```python
from build123d import *

# Parameters (mm, degrees)
CROQUIS1_R              = 8.15
CROQUIS1_R_2            = 1.6
SALIENTE_EXTRUIR1_DEPTH = 5
CROQUIS2_R              = 9.1
CORTAR_EXTRUIR1_DEPTH   = 1
CORTAR_EXTRUIR2_DEPTH   = 3
REDONDEO1_R             = 1
SALIENTE_EXTRUIR2_DEPTH = 46
CORTAR_EXTRUIR3_DEPTH   = 2
CORTAR_EXTRUIR4_REACH   = 103.242
CROQUIS6_R              = 2.6
CROQUIS6_W              = 5.6
CROQUIS6_H              = 3
CORTAR_EXTRUIR5_DEPTH   = 5
SALIENTE_EXTRUIR3_DEPTH = 46
CORTAR_EXTRUIR6_DEPTH   = 2
CORTAR_EXTRUIR7_REACH   = 103.242
CROQUIS10_R             = 2.6
CROQUIS10_W             = 5.6
CROQUIS10_H             = 3
CROQUIS11_R             = 1.6
CORTAR_EXTRUIR8_DEPTH   = 21
REDONDEO2_R             = 1


with BuildPart() as part:
    # Croquis1 → Saliente-Extruir1 (new body)
    with BuildSketch(Plane(origin=(0, 0, 0), x_dir=(1, 0, 0), z_dir=(0, 1, 0))):
        with BuildLine():
            Line((-30, -35), (30, -35))
            ThreePointArc((30, -35), (47.67766953, -27.67766953), (55, -10))
            Line((55, -10), (55, 15))
            ThreePointArc((55, 15), (49.142135624, 29.142135624), (35, 35))
            Line((35, 35), (-35, 35))
            ThreePointArc((-35, 35), (-49.142135624, 29.142135624), (-55, 15))
            Line((-55, 15), (-55, -10))
            ThreePointArc((-55, -10), (-47.67766953, -27.67766953), (-30, -35))
        make_face()
        with Locations(Location((39, 9, 0), (0, 0, 270))):
            Circle(CROQUIS1_R, mode=Mode.SUBTRACT)
        with Locations(Location((51.75, 12, 0), (0, 0, 270))):
            Circle(CROQUIS1_R_2, mode=Mode.SUBTRACT)
        with Locations(Location((51.75, -12, 0), (0, 0, 90))):
            Circle(CROQUIS1_R_2, mode=Mode.SUBTRACT)
        with Locations(Location((-51.75, -12, 0), (0, 0, 270))):
            Circle(CROQUIS1_R_2, mode=Mode.SUBTRACT)
        with Locations(Location((-51.75, 12, 0), (0, 0, 90))):
            Circle(CROQUIS1_R_2, mode=Mode.SUBTRACT)
        with Locations(Location((-39, 9, 0), (0, 0, 90))):
            Circle(CROQUIS1_R, mode=Mode.SUBTRACT)
        with BuildLine():
            Line((-10, -23), (10, -23))
            ThreePointArc((10, -23), (17.071067812, -20.071067812), (20, -13))
            Line((20, -13), (20, 13))
            ThreePointArc((20, 13), (17.071067812, 20.071067812), (10, 23))
            Line((10, 23), (-10, 23))
            ThreePointArc((-10, 23), (-17.071067812, 20.071067812), (-20, 13))
            Line((-20, 13), (-20, -13))
            ThreePointArc((-20, -13), (-17.071067812, -20.071067812), (-10, -23))
        make_face(mode=Mode.SUBTRACT)
    extrude(amount=SALIENTE_EXTRUIR1_DEPTH)

    # Croquis2 → Cortar-Extruir1 (cut)
    with BuildSketch(Plane(origin=(0, 5, 0), x_dir=(1, 0, 0), z_dir=(0, 1, 0))):
        with Locations(Location((39, 9, 0), (0, 0, 270))):
            Circle(CROQUIS2_R)
        with Locations(Location((-39, 9, 0), (0, 0, 90))):
            Circle(CROQUIS2_R)
    extrude(amount=-CORTAR_EXTRUIR1_DEPTH, mode=Mode.SUBTRACT)

    # Croquis3 → Cortar-Extruir2 (cut)
    with BuildSketch(Plane(origin=(0, 5, 0), x_dir=(1, 0, 0), z_dir=(0, 1, 0))):
        with BuildLine():
            Line((51.75, 15), (55, 15))
            Line((55, 15), (55, 9))
            Line((55, 9), (51.75, 9))
            ThreePointArc((51.75, 9), (48.75, 12), (51.75, 15))
        make_face()
        with BuildLine():
            Line((51.75, -15), (55, -15))
            Line((55, -15), (55, -9))
            Line((55, -9), (51.75, -9))
            ThreePointArc((51.75, -9), (48.75, -12), (51.75, -15))
        make_face()
        with BuildLine():
            Line((-51.75, -9), (-55, -9))
            Line((-55, -9), (-55, -15))
            Line((-55, -15), (-51.75, -15))
            ThreePointArc((-51.75, -15), (-48.75, -12), (-51.75, -9))
        make_face()
        with BuildLine():
            Line((-51.75, 15), (-55, 15))
            Line((-55, 15), (-55, 9))
            Line((-55, 9), (-51.75, 9))
            ThreePointArc((-51.75, 9), (-48.75, 12), (-51.75, 15))
        make_face()
    extrude(amount=-CORTAR_EXTRUIR2_DEPTH, mode=Mode.SUBTRACT)

    # Redondeo1
    redondeo1_edges = [part.edges().sort_by_distance(p)[0] for p in [
        (-55, 3.5, -9),
        (-55, 3.5, 9),
        (55, 3.5, 9),
        (55, 3.5, -9),
        (55, 3.5, -15),
        (-55, 3.5, -15),
        (54.494897428, 3.5, 15),
        (-54.494897428, 3.5, 15),
    ]]
    fillet(redondeo1_edges, radius=REDONDEO1_R)

    # Croquis4 → Saliente-Extruir2 (add)
    with BuildSketch(Plane(origin=(0, 5, 0), x_dir=(1, 0, 0), z_dir=(0, 1, 0))):
        with BuildLine():
            Line((-25, 35), (25, 35))
            Line((25, 35), (25, 28))
            ThreePointArc((25, 28), (23.535533906, 24.464466094), (20, 23))
            Line((20, 23), (-20, 23))
            ThreePointArc((-20, 23), (-23.535533906, 24.464466094), (-25, 28))
            Line((-25, 28), (-25, 35))
        make_face()
    extrude(amount=SALIENTE_EXTRUIR2_DEPTH)

    # Croquis5 → Cortar-Extruir3 (cut)
    with BuildSketch(Plane(origin=(0, 0, -35), x_dir=(-1, 0, 0), z_dir=(0, 0, -1))):
        with BuildLine():
            Line((-25, 51), (25, 51))
            Line((25, 51), (25, 17.708712153))
            ThreePointArc((25, 17.708712153), (22.970514841, 15.371172764), (20, 14.5))
            Line((20, 14.5), (-20, 14.5))
            ThreePointArc((-20, 14.5), (-22.970514841, 15.371172764), (-25, 17.708712153))
            Line((-25, 17.708712153), (-25, 51))
        make_face()
    extrude(amount=-CORTAR_EXTRUIR3_DEPTH, mode=Mode.SUBTRACT)

    # Cortar-Extruir4: up to this face of the body (flat: up to its plane)
    cortar_extruir4_end = Plane(part.part.faces().sort_by_distance((0, 26.68556701, -23))[0])
    # Croquis6 → Cortar-Extruir4 (cut, up to the picked face)
    with BuildSketch(Plane(origin=(0, 0, -33), x_dir=(-1, 0, 0), z_dir=(0, 0, -1)), mode=Mode.PRIVATE) as cortar_extruir4_sk1:
        with Locations((-20, 20)):
            Circle(CROQUIS6_R)
    cortar_extruir4_tool1 = split(extrude(cortar_extruir4_sk1.sketch, amount=-CORTAR_EXTRUIR4_REACH, mode=Mode.PRIVATE), bisect_by=cortar_extruir4_end, keep=Keep.BOTH, mode=Mode.PRIVATE)
    # Croquis6 → Cortar-Extruir4 (cut, up to the picked face)
    with BuildSketch(Plane(origin=(0, 0, -33), x_dir=(-1, 0, 0), z_dir=(0, 0, -1)), mode=Mode.PRIVATE) as cortar_extruir4_sk2:
        with Locations(Location((20, 20, 0), (0, 0, 90))):
            Circle(CROQUIS6_R)
    cortar_extruir4_tool2 = split(extrude(cortar_extruir4_sk2.sketch, amount=-CORTAR_EXTRUIR4_REACH, mode=Mode.PRIVATE), bisect_by=cortar_extruir4_end, keep=Keep.BOTH, mode=Mode.PRIVATE)
    # Croquis6 → Cortar-Extruir4 (cut, up to the picked face)
    with BuildSketch(Plane(origin=(0, 0, -33), x_dir=(-1, 0, 0), z_dir=(0, 0, -1)), mode=Mode.PRIVATE) as cortar_extruir4_sk3:
        with Locations((-20, 44.5)):
            Rectangle(CROQUIS6_W, CROQUIS6_H)
    cortar_extruir4_tool3 = split(extrude(cortar_extruir4_sk3.sketch, amount=-CORTAR_EXTRUIR4_REACH, mode=Mode.PRIVATE), bisect_by=cortar_extruir4_end, keep=Keep.BOTH, mode=Mode.PRIVATE)
    # Croquis6 → Cortar-Extruir4 (cut, up to the picked face)
    with BuildSketch(Plane(origin=(0, 0, -33), x_dir=(-1, 0, 0), z_dir=(0, 0, -1)), mode=Mode.PRIVATE) as cortar_extruir4_sk4:
        with Locations((20, 44.5)):
            Rectangle(CROQUIS6_W, CROQUIS6_H)
    cortar_extruir4_tool4 = split(extrude(cortar_extruir4_sk4.sketch, amount=-CORTAR_EXTRUIR4_REACH, mode=Mode.PRIVATE), bisect_by=cortar_extruir4_end, keep=Keep.BOTH, mode=Mode.PRIVATE)
    add(cortar_extruir4_tool1.solids().sort_by(Axis((20, 20, -33), (0, 0, 1)))[0], mode=Mode.SUBTRACT)
    add(cortar_extruir4_tool2.solids().sort_by(Axis((-20, 20, -33), (0, 0, 1)))[0], mode=Mode.SUBTRACT)
    add(cortar_extruir4_tool3.solids().sort_by(Axis((20, 44.5, -33), (0, 0, 1)))[0], mode=Mode.SUBTRACT)
    add(cortar_extruir4_tool4.solids().sort_by(Axis((-20, 44.5, -33), (0, 0, 1)))[0], mode=Mode.SUBTRACT)

    # Croquis7 → Cortar-Extruir5 (cut)
    with BuildSketch(Plane.XY.offset(-23)):
        Polygon((-20, 24.7), (-24.070319398, 22.35), (-24.070319398, 17.65), (-20, 15.3), (-15.929680602, 17.65), (-15.929680602, 22.35), align=None)
        Polygon((15.929680602, 22.35), (20, 24.7), (24.070319398, 22.35), (24.070319398, 17.65), (20, 15.3), (15.929680602, 17.65), align=None)
    extrude(amount=-CORTAR_EXTRUIR5_DEPTH, mode=Mode.SUBTRACT)

    # Croquis8 → Saliente-Extruir3 (add)
    with BuildSketch(Plane(origin=(0, 5, 0), x_dir=(1, 0, 0), z_dir=(0, 1, 0))):
        with BuildLine():
            Line((-10, -35), (10, -35))
            Line((10, -35), (10, -28))
            ThreePointArc((10, -28), (8.535533906, -24.464466094), (5, -23))
            Line((5, -23), (-5, -23))
            ThreePointArc((-5, -23), (-8.535533906, -24.464466094), (-10, -28))
            Line((-10, -28), (-10, -35))
        make_face()
    extrude(amount=SALIENTE_EXTRUIR3_DEPTH)

    # Croquis9 → Cortar-Extruir6 (cut)
    with BuildSketch(Plane.XY.offset(35)):
        with BuildLine():
            Line((10, 17.708712153), (10, 51))
            Line((10, 51), (-10, 51))
            Line((-10, 51), (-10, 17.708712153))
            ThreePointArc((-10, 17.708712153), (-7.970514841, 15.371172764), (-5, 14.5))
            Line((-5, 14.5), (5, 14.5))
            ThreePointArc((5, 14.5), (7.970514841, 15.371172764), (10, 17.708712153))
        make_face()
    extrude(amount=-CORTAR_EXTRUIR6_DEPTH, mode=Mode.SUBTRACT)

    # Cortar-Extruir7: up to this face of the body (flat: up to its plane)
    cortar_extruir7_end = Plane(part.part.faces().sort_by_distance((0, 23.446428571, 23))[0])
    # Croquis10 → Cortar-Extruir7 (cut, up to the picked face)
    with BuildSketch(Plane.XY.offset(33), mode=Mode.PRIVATE) as cortar_extruir7_sk1:
        with Locations((-5, 20)):
            Circle(CROQUIS10_R)
    cortar_extruir7_tool1 = split(extrude(cortar_extruir7_sk1.sketch, amount=-CORTAR_EXTRUIR7_REACH, mode=Mode.PRIVATE), bisect_by=cortar_extruir7_end, keep=Keep.BOTH, mode=Mode.PRIVATE)
    # Croquis10 → Cortar-Extruir7 (cut, up to the picked face)
    with BuildSketch(Plane.XY.offset(33), mode=Mode.PRIVATE) as cortar_extruir7_sk2:
        with Locations(Location((5, 20, 0), (0, 0, 90))):
            Circle(CROQUIS10_R)
    cortar_extruir7_tool2 = split(extrude(cortar_extruir7_sk2.sketch, amount=-CORTAR_EXTRUIR7_REACH, mode=Mode.PRIVATE), bisect_by=cortar_extruir7_end, keep=Keep.BOTH, mode=Mode.PRIVATE)
    # Croquis10 → Cortar-Extruir7 (cut, up to the picked face)
    with BuildSketch(Plane.XY.offset(33), mode=Mode.PRIVATE) as cortar_extruir7_sk3:
        with Locations((-5, 44.5)):
            Rectangle(CROQUIS10_W, CROQUIS10_H)
    cortar_extruir7_tool3 = split(extrude(cortar_extruir7_sk3.sketch, amount=-CORTAR_EXTRUIR7_REACH, mode=Mode.PRIVATE), bisect_by=cortar_extruir7_end, keep=Keep.BOTH, mode=Mode.PRIVATE)
    # Croquis10 → Cortar-Extruir7 (cut, up to the picked face)
    with BuildSketch(Plane.XY.offset(33), mode=Mode.PRIVATE) as cortar_extruir7_sk4:
        with Locations((5, 44.5)):
            Rectangle(CROQUIS10_W, CROQUIS10_H)
    cortar_extruir7_tool4 = split(extrude(cortar_extruir7_sk4.sketch, amount=-CORTAR_EXTRUIR7_REACH, mode=Mode.PRIVATE), bisect_by=cortar_extruir7_end, keep=Keep.BOTH, mode=Mode.PRIVATE)
    add(cortar_extruir7_tool1.solids().sort_by(Axis((-5, 20, 33), (0, 0, -1)))[0], mode=Mode.SUBTRACT)
    add(cortar_extruir7_tool2.solids().sort_by(Axis((5, 20, 33), (0, 0, -1)))[0], mode=Mode.SUBTRACT)
    add(cortar_extruir7_tool3.solids().sort_by(Axis((-5, 44.5, 33), (0, 0, -1)))[0], mode=Mode.SUBTRACT)
    add(cortar_extruir7_tool4.solids().sort_by(Axis((5, 44.5, 33), (0, 0, -1)))[0], mode=Mode.SUBTRACT)

    # Croquis11 → Cortar-Extruir8 (cut)
    with BuildSketch(Plane(origin=(0, 51, 0), x_dir=(1, 0, 0), z_dir=(0, 1, 0))):
        with Locations(Location((-5, -28, 0), (0, 0, 270))):
            Circle(CROQUIS11_R)
        with Locations(Location((-20, 28, 0), (0, 0, 270))):
            Circle(CROQUIS11_R)
        with Locations(Location((5, -28, 0), (0, 0, 270))):
            Circle(CROQUIS11_R)
        with Locations(Location((20, 28, 0), (0, 0, 270))):
            Circle(CROQUIS11_R)
    extrude(amount=-CORTAR_EXTRUIR8_DEPTH, mode=Mode.SUBTRACT)

    # Redondeo2
    redondeo2_edges = [part.edges().sort_by_distance(p)[0] for p in [
        (25, 17.708712153, -34),
        (-25, 17.708712153, -34),
        (10, 17.708712153, 34),
        (-10, 17.708712153, 34),
    ]]
    fillet(redondeo2_edges, radius=REDONDEO2_R)


solid = part.part
```
Work out the finished part from the listing and answer in its coordinate system (mm). A direction names the side the tool comes from. Give positions to 0.01 mm unless a question says otherwise; leave off trailing zeros. Order: outer loops, then holes, each group sorted by start corner. A loop starts at its lowest first (then second) coordinate and runs counter-clockwise, first axis right, second up.
1. For faces 1 (the flat face through (20, 2, 0)), 2 (the flat face through (-17.99, 16.46, -25.46)), 3 (the cylindrical face through (-48.023, 4.507, -7.815)), 4 (the flat face through (-18.7, 46, -29.2)), determine the directions among +Z, -Z, +X, -X, +Y, -Y from which every point of the face is accessible in a straight line to the end or side of a thin tool.
Result sheet:
face 1: +Y, -Y
face 2: +Z
face 3: +Y
face 4: +Z, -Z
2. Straight lines are drawn through the part: L1, parallel to X at y = 38, z = 28; L2, parallel to X at y = 20, z = 29; L3, parallel to Y at x = 20, z = -29.3. For each, find the intervals that lie inside material, in ascending order.
Result sheet:
L1: x = -10 to -6.6, -3.4 to 3.4, 6.6 to 10
L2: x = -10 to -7.6, -2.4 to 2.4, 7.6 to 10
L3: y = 0 to 17.4, 22.6 to 30
3. Section A-A, the plane y = 39 is taken. Determine the outline of the cut face in (x, z), and give its area (3 significant figures).
Result sheet:
outline: (-25, -33) - (25, -33) - (25, -28) arc R5 ccw to (20, -23) - (-20, -23) arc R5 ccw to (-25, -28) - close; (-10, 28) arc R5 ccw to (-5, 23) - (5, 23) arc R5 ccw to (10, 28) - (10, 33) - (-10, 33) - close; hole circle Ø3.2 at (-20, -28); hole circle Ø3.2 at (-5, 28); hole circle Ø3.2 at (5, 28); hole circle Ø3.2 at (20, -28)
area: 646 mm2
4. Section B-B, the plane y = 27 is taken. Determine the outline of the cut face in (x, z), and give its area (3 significant figures).
Result sheet:
outline: (-25, -33) - (25, -33) - (25, -28) arc R5 ccw to (20, -23) - (-20, -23) arc R5 ccw to (-25, -28) - close; (-10, 28) arc R5 ccw to (-5, 23) - (5, 23) arc R5 ccw to (10, 28) - (10, 33) - (-10, 33) - close
area: 679 mm2
5. The mould has two halves that part along X. Classify faces 5 (the flat face through (20, 30, -28)), 6 (the flat face through (-20, 2, 0)), 7 (the flat face through (-1, 0, -24)), 8 (the cylindrical face through (47.482, 2.465, 27.871)): released by +X, released by -X, zero draft, split by the parting line, or undercut.
Result sheet:
face 5: undercut
face 6: undercut
face 7: zero draft
face 8: released by +X
6. Section C-C, the plane z = -31 is taken. Determine the outline of the cut face in (x, y), and give its area (3 significant figures).
Result sheet:
outline: (-47, 0) - (47, 0) - (47, 5) - (25, 5) - (25, 51) - (-25, 51) - (-25, 5) - (-47, 5) - close; hole (-22.8, 43) - (-17.2, 43) - (-17.2, 46) - (-22.8, 46) - close; hole circle Ø5.2 at (-20, 20); hole (17.2, 43) - (22.8, 43) - (22.8, 46) - (17.2, 46) - close; hole circle Ø5.2 at (20, 20)
area: 2,690 mm2
7. Section D-D, the plane x = 43.5 is taken. Determine the outline of the cut face in (y, z), and give its area (3 significant figures).
Result sheet:
outline: (0, -33.1) - (5, -33.1) - (5, -16.91) - (4, -16.91) - (4, -15.8) - (0, -15.8) - close; (0, -2.2) - (4, -2.2) - (4, -1.09) - (5, -1.09) - (5, 31.04) - (0, 31.04) - close
area: 251 mm2
8. Each of these flat-tipped pins is pushed along its axis until it touches: P1, Ø0.9, axis at y = 45, z = -27.5, coming from the +X side; P2, Ø4, axis at y = 20, z = -25, coming from the -X side; P3, Ø4, axis at x = -51.75, z = 12, coming from the +Y side. Where does it stop, or does it pass through?
Result sheet:
P1: stops at x = 25
P2: stops at x = -24.9
P3: stops at y = 2
